Work out the finished part from the listing and answer in its coordinate system (mm). A direction names the side the tool comes from. Give positions to 0.01 mm unless a question says otherwise; leave off trailing zeros. Loops run counter-clockwise (first coordinate to the right, second up) from the corner with the lowest first, then second, coordinate; pieces in that order, holes last. Notation, with made-up numbers: M -30,-4 L 5,-4 A15 ccw 5,22 Z; hole C 70,15 d5. An arc over 180 degrees is marked long. Write item = value, one per line. Start each with the question number.
1. Section B-B on z = -1.25 is taken. Determine the outline of the cut face in (x, y), plus the area to 3 significant figures.
2. Section C-C on x = 0 is taken. Determine the outline of the cut face in (y, z), plus the area to 3 significant figures.
3. The mould has two halves that part along Y. Classify faces 5 (the face through (-8, 12, 11)), 6 (the face through (-4, 8, -3)), 7 (the face through (0, 19, -1)), 8 (the face through (-6, 17, -1)): released by +Y, released by -Y, zero draft, split by the parting line, or undercut.
4. For faces 1 (the face through (0, 1, 17)), 2 (the face through (0, 2, 1)), 3 (the face through (-2.75, 0, 9)), 4 (the face through (0, 16, -1)), determine the directions among +Z, -Z, +X, -X, +Y, -Y from which every point of the face is accessible in a straight line to the end or side of a thin tool.
5. Section A-A on y = 7.75 is taken. Determine the outline of the cut face in (x, z), plus the area to 3 significant figures.
6. Flat-ended cylindrical pins translate along their axes: pin 1 Ø2 at (x, z) = (1.5, 16.5) entering from +Y; pin 2 Ø1.2 at (x, z) = (3, 0) entering from -Y; pin 3 Ø1.5 at (x, y) = (-0.5, 17) entering from -Z. Find the tip coordinate at first contact, or state that the pin passes through.
7. Consider L1, parallel to Z at x = 5.5, y = -0.75; L2, parallel to X at y = 11, z = 8.75; L3, parallel to X at y = 0.5, z = 7.75. Determine where each line is inside the solid, lowest interval first. Write a range as [from, to].
8. Section D-D on z = 10 is taken. Determine the outline of the cut face in (x, y), plus the area to 3 significant figures.
Autodesk Inventor part; units mm, degrees
ref_plane "YZ Plane" through (0, 0, 0) normal (1, 0, 0) x (0, 1, 0)
ref_plane "XZ Plane" through (0, 0, 0) normal (0, 1, 0) x (-1, 0, 0)
ref_plane "XY Plane" through (0, 0, 0) normal (0, 0, 1) x (1, 0, 0)
sketch "Sketch_1" plane through (0, 0, 0) normal (1, 0, 0) x (0, 1, 0)
  line L0 (0, 20) -> (0, 0)
  line L1 (0, 0) -> (20, 0)
  line L2 (20, 0) -> (20, 3)
  line L3 (20, 3) -> (3, 20)
  line L4 (3, 20) -> (0, 20)
  dimension "d35" = 20
  dimension "d36" = 20
  dimension "d37" = 17
  dimension "d38" = 3
extrude "Extrusion1" add sketch "Sketch_1" along normal mid plane 17
sketch "Sketch_2" plane through (0, 0, 0) normal (1, 0, 0) x (0, 1, 0)
  line L0 (3, 20) -> (3, 3.5)
  arc A0 (3, 3.5) -> (3.5, 3) centre (3.5, 3.5) ccw
  line L1 (3.5, 3) -> (20, 3)
  line L2 (20, 3) -> (3, 20)
extrude "Extrusion2" cut sketch "Sketch_2" along normal mid plane 13
sketch "Sketch_3" plane through (0, 0, 0) normal (1, 0, 0) x (0, 1, 0)
  line L0 (0, 3) -> (0, 0)
  line L1 (0, 0) -> (3, 0)
  line L2 (3, 0) -> (3, 1)
  line L3 (3, 1) -> (1, 1)
  line L4 (1, 1) -> (1, 3)
  line L5 (1, 3) -> (0, 3)
extrude "Extrusion3" cut sketch "Sketch_3" along normal mid plane 12
sketch "Sketch_4" plane through (0, 0, 0) normal (1, 0, 0) x (0, 1, 0)
  line L0 (0, 19) -> (0, 16)
  line L1 (0, 16) -> (1, 16)
  line L2 (1, 16) -> (1, 19)
  line L3 (1, 19) -> (0, 19)
extrude "Extrusion4" cut sketch "Sketch_4" along normal mid plane 12
sketch "Sketch_5" plane through (0, 0, 0) normal (1, 0, 0) x (0, 1, 0)
  line L0 (16, 1) -> (16, 0)
  line L1 (16, 0) -> (19, 0)
  line L2 (19, 0) -> (19, 1)
  line L3 (19, 1) -> (16, 1)
extrude "Extrusion5" cut sketch "Sketch_5" along normal mid plane 12
move faces "Move1" translate (0, 0, -3) faces at (-2, 7.3333, 0) (-2, 0, 11.6667)
move faces "Move2" translate (0, -3, 0) faces at (-2, 0, 7.3333)
sketch "Sketch8" plane through (-8.5, -3, 20) normal (0, -1, 0) x (1, 0, 0)
  line L0 (8.5, -9) -> (8.5, -13) construction
  line L1 (5.75, -9) -> (5.75, -13)
  line L2 (11.25, -13) -> (11.25, -9)
  arc A0 (11.25, -9) -> (5.75, -9) centre (8.5, -9) ccw
  arc A1 (5.75, -13) -> (11.25, -13) centre (8.5, -13) ccw
  line L3 (14.5, -23) -> (2.5, -23)
  line L4 (17, 0) -> (17, -23)
  point P0 (8.5, -20)
  point P1 (8.5, -11)
  dimension "d23" = 2
  dimension "d24" = 5.5
  dimension "d25" = 12
  dimension "d32" = 8.5
extrude "Extrusion8" cut sketch "Sketch8" against normal through all
sketch "Sketch9" plane through (8.5, 20, -3) normal (0, 0, -1) x (-1, 0, 0)
  line L0 (8.5, -9) -> (8.5, -13) construction
  line L1 (5.75, -9) -> (5.75, -13)
  line L2 (11.25, -13) -> (11.25, -9)
  arc A0 (11.25, -9) -> (5.75, -9) centre (8.5, -9) ccw
  arc A1 (5.75, -13) -> (11.25, -13) centre (8.5, -13) ccw
  line L3 (17, -23) -> (14.5, -23)
  line L4 (0, -23) -> (0, 0)
  point P0 (8.5, -20)
  point P1 (8.5, -11)
  dimension "d28" = 2
  dimension "d29" = 5.5
  dimension "d30" = 12
  dimension "d31" = 8.5
extrude "Extrusion9" cut sketch "Sketch9" against normal through all
properties part number "14056_m"
Verdict:
q1.outline = M -8.5,-3 L -6,-3 L -6,3 L 6,3 L 6,-3 L 8.5,-3 L 8.5,20 L -8.5,20 Z; hole M -6,16 L 6,16 L 6,19 L -6,19 Z; hole M -2.75,7 A2.75 ccw 2.75,7 L 2.75,11 A2.75 ccw -2.75,11 Z
q1.area = 237 mm2
q2.outline = M -3,3 L 1,3 L 1,1 L 3,1 L 3,-3 L 4.25,-3 L 4.25,3 L 3.5,3 A0.5 cw 3,3.5 L 3,4.25 L -3,4.25 Z; M -3,13.75 L 3,13.75 L 3,20 L -3,20 L -3,19 L 1,19 L 1,16 L -3,16 Z; M 13.75,-3 L 16,-3 L 16,1 L 19,1 L 19,-3 L 20,-3 L 20,3 L 13.75,3 Z
q2.area = 70.1 mm2
q3.face_5 = released by +Y
q3.face_6 = zero draft
q3.face_7 = undercut
q3.face_8 = undercut
q4.face_1 = -Y
q4.face_2 = -Z, -Y
q4.face_3 = +Y, -Y
q4.face_4 = -Z
q5.outline = M -8.5,-3 L -2.75,-3 L -2.75,3 L -6.5,3 L -6.5,15.25 L -8.5,15.25 Z; M 2.75,-3 L 8.5,-3 L 8.5,15.25 L 6.5,15.25 L 6.5,3 L 2.75,3 Z
q5.area = 118 mm2
q6.pin_1 = 3
q6.pin_2 = 3
q6.pin_3 = 1
q7.L1 = [3, 16], [19, 20]
q7.L2 = [-8.5, -6.5], [6.5, 8.5]
q7.L3 = [-8.5, -2.75], [2.75, 8.5]
q8.outline = M -8.5,-3 L -2.75,-3 L -2.75,3 L -6.5,3 L -6.5,13 L -8.5,13 Z; M 2.75,-3 L 8.5,-3 L 8.5,13 L 6.5,13 L 6.5,3 L 2.75,3 Z
q8.area = 109 mm2
